The listing builds one solid part. Answer for the finished solid, in the listing's coordinates (mm). Face numbers are marked on the shaded views. A direction names the side the tool comes from. Coordinates: 2 decimals unless noted, no trailing zeros. Order: outer loops, then holes, each group sorted by start corner. A loop starts at its lowest first (then second) coordinate and runs counter-clockwise, first axis right, second up. Notation, with made-up numbers: (88, 66) -> (147, 66) arc R22 ccw to (147, 85) -> close; hole circle Ø9 at (44, -29.75). An arc over 180 degrees is marked (long way). Write each question's results on one line, items separated by ' | '. Start each with the question number.
(1) The part is cut by section D-D, the plane y = 42. Give the vertices of the cut face in (x, z), then the cut area to 3 significant figures.
(2) Straight lines are drawn through the part: L1, parallel to X at y = 37.5, z = 6.25; L2, parallel to Z at x = 6, y = 26; L3, parallel to Y at x = 23, z = 10.5. For each, find the intervals that lie inside material, in ascending order.
(3) Determine the mould class of the marked faces 1, 2 and 3 for opening direction X: +X half, -X half, draft (parallel to the pull), parting line (faces both ways), or undercut.
(4) A tool of negligible diameter and unlimited length cuts with its end or side. For the marked faces 4, 5 and 6, from which of +Z, -Z, +X, -X, +Y, -Y can it reach the whole face along a straight path? Write none if from no direction.
(5) Given pin 1 (10 mm diameter, centred on y = 30, z = -10, fed in from +X); pin 2 (6 mm diameter, centred on x = -6.25, z = 6.25, fed in from +Y); pin 3 (12 mm diameter, centred on x = -19.5, y = 40.5, fed in from -Z); pin 4 (3.5 mm diameter, centred on x = -20, z = 10.5, fed in from -Y), each flat-ended and moving along its own axis, determine where each tip first touches the part or whether it passes through.
(6) The part is cut by section A-A, the plane x = -6.25. Give the vertices of the cut face in (y, z).
(7) The part is cut by section C-C, the plane z = -6.25. Give the vertices of the cut face in (x, y), then the cut area to 3 significant figures.
(8) The part is cut by section B-B, the plane y = 11. Give the vertices of the cut face in (x, z), then the cut area to 3 significant figures.
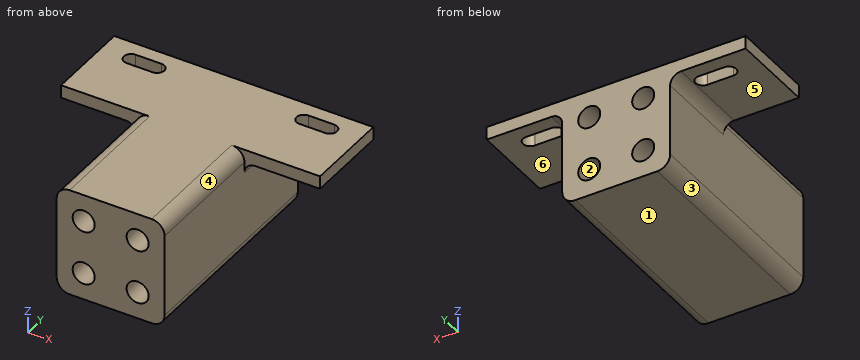
```python
from build123d import *

# Parameters (mm, degrees)
SKETCH_1_R          = 2.55
EXTRUDE_1_DEPTH     = 30
SKETCH_2_R          = 2.55
EXTRUDE_2_DEPTH     = 20
CUT_EXTRUDE_1_DEPTH = 20
FILLET_1_R          = 2.5


with BuildPart() as part:
    # 草图1 → 凸台-拉伸1 (new body)
    with BuildSketch(Plane(origin=(0, 0, 0), x_dir=(1, 0, 0), z_dir=(0, 1, 0))):
        with BuildLine():
            Line((-9.5, 12.5), (9.5, 12.5))
            ThreePointArc((9.5, 12.5), (11.621320344, 11.621320344), (12.5, 9.5))
            Line((12.5, 9.5), (12.5, -9.5))
            ThreePointArc((12.5, -9.5), (11.621320344, -11.621320344), (9.5, -12.5))
            Line((9.5, -12.5), (-9.5, -12.5))
            ThreePointArc((-9.5, -12.5), (-11.621320344, -11.621320344), (-12.5, -9.5))
            Line((-12.5, -9.5), (-12.5, 9.5))
            ThreePointArc((-12.5, 9.5), (-11.621320344, 11.621320344), (-9.5, 12.5))
        make_face()
        with Locations(Location((6.25, 6.25, 0), (0, 0, 270))):
            Circle(SKETCH_1_R, mode=Mode.SUBTRACT)
        with Locations(Location((-6.25, 6.25, 0), (0, 0, 270))):
            Circle(SKETCH_1_R, mode=Mode.SUBTRACT)
        with Locations(Location((-6.25, -6.25, 0), (0, 0, 270))):
            Circle(SKETCH_1_R, mode=Mode.SUBTRACT)
        with Locations(Location((6.25, -6.25, 0), (0, 0, 270))):
            Circle(SKETCH_1_R, mode=Mode.SUBTRACT)
    extrude(amount=EXTRUDE_1_DEPTH)

    # 草图2 → 凸台-拉伸2 (add)
    with BuildSketch(Plane(origin=(0, 30, 0), x_dir=(1, 0, 0), z_dir=(0, 1, 0))):
        with BuildLine():
            Line((-9.5, -12.5), (-30, -12.5))
            Line((-30, -12.5), (-30, -9.5))
            Line((-30, -9.5), (-12.5, -9.5))
            Line((-12.5, -9.5), (-12.5, 9.5))
            ThreePointArc((-12.5, 9.5), (-11.621320344, 11.621320344), (-9.5, 12.5))
            Line((-9.5, 12.5), (9.5, 12.5))
            ThreePointArc((9.5, 12.5), (11.621320344, 11.621320344), (12.5, 9.5))
            Line((12.5, 9.5), (12.5, -9.5))
            Line((12.5, -9.5), (30, -9.5))
            Line((30, -9.5), (30, -12.5))
            Line((30, -12.5), (9.5, -12.5))
            Line((9.5, -12.5), (-9.5, -12.5))
        make_face()
        with Locations(Location((-6.25, 6.25, 0), (0, 0, 270))):
            Circle(SKETCH_2_R, mode=Mode.SUBTRACT)
        with Locations(Location((6.25, 6.25, 0), (0, 0, 270))):
            Circle(SKETCH_2_R, mode=Mode.SUBTRACT)
        with Locations(Location((-6.25, -6.25, 0), (0, 0, 270))):
            Circle(SKETCH_2_R, mode=Mode.SUBTRACT)
        with Locations(Location((6.25, -6.25, 0), (0, 0, 270))):
            Circle(SKETCH_2_R, mode=Mode.SUBTRACT)
    extrude(amount=EXTRUDE_2_DEPTH)

    # 草图3 → 切除-拉伸1 (cut)
    with BuildSketch(Plane(origin=(0, 0, 9.5), x_dir=(-1, 0, 0), z_dir=(0, 0, -1))):
        with BuildLine():
            Line((-23, 46.7), (-17, 46.7))
            ThreePointArc((-17, 46.7), (-15.3, 45), (-17, 43.3))
            Line((-17, 43.3), (-23, 43.3))
            ThreePointArc((-23, 43.3), (-24.7, 45), (-23, 46.7))
        make_face()
        with BuildLine():
            Line((23, 43.3), (17, 43.3))
            ThreePointArc((17, 43.3), (15.3, 45), (17, 46.7))
            Line((17, 46.7), (23, 46.7))
            ThreePointArc((23, 46.7), (24.7, 45), (23, 43.3))
        make_face()
    extrude(amount=-CUT_EXTRUDE_1_DEPTH, mode=Mode.SUBTRACT)

    # 圆角1
    fillet_1_edges = [part.edges().sort_by_distance(p)[0] for p in [
        (12.5, 40, 9.5),
        (-12.5, 40, 9.5),
    ]]
    fillet(fillet_1_edges, radius=FILLET_1_R)


solid = part.part
```
Established:
1) outline: (-30, 9.5) -> (-15, 9.5) arc R2.5 cw to (-12.5, 7) -> (-12.5, -9.5) arc R3 ccw to (-9.5, -12.5) -> (9.5, -12.5) arc R3 ccw to (12.5, -9.5) -> (12.5, 7) arc R2.5 cw to (15, 9.5) -> (30, 9.5) -> (30, 12.5) -> (-30, 12.5) -> close; hole circle Ø5.1 at (-6.25, -6.25); hole circle Ø5.1 at (-6.25, 6.25); hole circle Ø5.1 at (6.25, -6.25); hole circle Ø5.1 at (6.25, 6.25) | area: 647 mm^2
2) L1: x = -12.5 to -8.8, -3.7 to 3.7, 8.8 to 12.5 | L2: z = -12.5 to -8.79, -3.71 to 3.71, 8.79 to 12.5 | L3: y = 30 to 43.3, 46.7 to 50
3) face 1: draft | face 2: undercut | face 3: -X half
4) face 4: +Z, +X, -Y | face 5: -Z, -X, +Y, -Y | face 6: -Z, +X, +Y, -Y
5) pin 1: stops at x = 12.5 | pin 2: stops at y = 50 | pin 3: stops at z = 9 | pin 4: stops at y = 30
6) outline: (0, -12.5) -> (50, -12.5) -> (50, -8.8) -> (0, -8.8) -> close; (0, -3.7) -> (50, -3.7) -> (50, 3.7) -> (0, 3.7) -> close; (0, 8.8) -> (50, 8.8) -> (50, 12.5) -> (0, 12.5) -> close
7) outline: (-12.5, 0) -> (-8.8, 0) -> (-8.8, 50) -> (-12.5, 50) -> close; (-3.7, 0) -> (3.7, 0) -> (3.7, 50) -> (-3.7, 50) -> close; (8.8, 0) -> (12.5, 0) -> (12.5, 50) -> (8.8, 50) -> close | area: 740 mm^2
8) outline: (-12.5, -9.5) arc R3 ccw to (-9.5, -12.5) -> (9.5, -12.5) arc R3 ccw to (12.5, -9.5) -> (12.5, 9.5) arc R3 ccw to (9.5, 12.5) -> (-9.5, 12.5) arc R3 ccw to (-12.5, 9.5) -> close; hole circle Ø5.1 at (-6.25, -6.25); hole circle Ø5.1 at (-6.25, 6.25); hole circle Ø5.1 at (6.25, -6.25); hole circle Ø5.1 at (6.25, 6.25) | area: 536 mm^2
